Source: CAD feature listing. Evaluate the final solid. Frame: model axes, mm. Give positions to 0.01 mm unless a question says otherwise; leave off trailing zeros. Write each loop counter-clockwise with the first axis right and the second up, starting at its lowest first coordinate (ties: lowest second). Pieces come first, ordered by that corner, then holes. Notation, with made-up numbers: M 20.5,35 L 57.5,35 A19 ccw 57.5,54 Z; hole C -4.5,-27 d1. An arc over 180 degrees is marked long. Return JSON: item names as keys, results as strings.
Autodesk Inventor part; units mm, degrees
ref_plane "YZ Plane" through (0, 0, 0) normal (1, 0, 0) x (0, 1, 0)
ref_plane "XZ Plane" through (0, 0, 0) normal (0, 1, 0) x (-1, 0, 0)
ref_plane "XY Plane" through (0, 0, 0) normal (0, 0, 1) x (1, 0, 0)
sketch "Skizze1" plane through (0, 0, 0) normal (0, 0, 1) x (1, 0, 0)
  line L0 (0, -7) -> (0, 7)
  line L1 (-7, 0) -> (7, 0)
  circle A0 centre (0, 0) radius 5
  dimension "d0" = 10
extrude "Extrusion1" add sketch "Skizze1" along normal mid plane 500
chamfer "Fase1" distance 0.2 angle 45 1 edges at (-5, 0, 250)
chamfer "Fase2" distance 0.2 angle 45 1 edges at (-5, 0, -250)
properties part number "10mm_Alu_Linearwelle_500mm" material "Aluminum 6061-AHC"
1) Line query: line 1 (X direction, y = -1.5, z = -8); line 2 (X direction, y = 0.5, z = -171.5); line 3 (Y direction, x = 0.25, z = -179). Output: solid intervals per line, ascending. Write a range as [from, to].
Numbers:
{"line 1": "x = [-4.77, 4.77]", "line 2": "x = [-4.97, 4.97]", "line 3": "y = [-4.99, 4.99]"}
2) Contact query for a flat-ended pin moving along its axis: pin 1 Ø1 at (y, z) = (-1, -74) entering from -X. Output: stop coordinate, or through.
Numbers:
{"pin 1": "stops at x = -4.97"}
3) Cut plane A-A, the plane z = 199.5. Return the cut outline in (x, y).
Numbers:
{"outline": "C 0,0 d10"}
